from build123d import *

# Parameters (mm, degrees)
F2_SIZE = 0.25
F3_SIZE = 0.25


with BuildPart() as f1:
    # F0 (on Right) → F1 (revolve)
    with BuildSketch(Plane.YZ):
        Polygon((17.9, 6), (16.4, 4.5), (16.4, 0), (18.9, 0), (20.9, 2), (20.9, 6), align=None)
    revolve(axis=Axis((0, 0, 6.363279), (0, 0, 1)))

    # F2
    f2_edges = [f1.edges().sort_by_distance(p)[0] for p in [
        (0, -20.9, 6),
    ]]
    chamfer(f2_edges, length=F2_SIZE)

    # F3
    f3_edges = [f1.edges().sort_by_distance(p)[0] for p in [
        (0, -16.4, 0),
    ]]
    chamfer(f3_edges, length=F3_SIZE)


solid = f1.part
Verification items for the finished model (mm, model axes). Coordinates: 2 decimals unless noted, no trailing zeros. Order: outer loops, then holes, each group sorted by start corner. A loop starts at its lowest first (then second) coordinate and runs counter-clockwise, first axis right, second up.
1. Sectioned sample at A-A, the plane y = 0. Record the cut outline in (x, z).
Results found:
outline: (-20.9, 2) - (-18.9, 0) - (-16.65, 0) - (-16.4, 0.25) - (-16.4, 4.5) - (-17.9, 6) - (-20.65, 6) - (-20.9, 5.75) - close; (16.4, 0.25) - (16.65, 0) - (18.9, 0) - (20.9, 2) - (20.9, 5.75) - (20.65, 6) - (17.9, 6) - (16.4, 4.5) - close
2. Sectioned sample at C-C, the plane z = 5. Record the cut outline in (x, y), and give its area (3 significant figures).
Results found:
outline: circle Ø41.8 at (0, 0); hole circle Ø33.8 at (0, 0)
area: 475 mm2
3. Release check for a two-part mould opening along X. For faces 1 (the face through (-18.5, -0.1, 6)), 2 (the face through (-18.863, -2.477, 0.125)), 3 (the face through (-16.26, -2.13, 2.35)) record: +X half, -X half, draft (parallel to the pull), parting line (faces both ways), or undercut.
Results found:
face 1: draft
face 2: parting line
face 3: undercut
4. Go/stop test with a flat-tipped pin: pin 1 Ø1.5 at (y, z) = (15.5, 4.5) entering from -X. Record where the tip stops, or that it passes through.
Results found:
pin 1: stops at x = -14.81
5. Scan lines: line 1 (Y direction, x = 0, z = 2.45); line 2 (Y direction, x = 11.5, z = 5.1). Record each from-to range of solid material in increasing order.
Results found:
line 1: y = -20.9 to -16.4, 16.4 to 20.9
line 2: y = -17.45 to -12.52, 12.52 to 17.45
